Could you check a few things on this model? Use its own coordinates, in mm. Face numbers are marked on the shaded views. A direction names the side the tool comes from. Give positions to 0.01 mm unless a question says otherwise; leave off trailing zeros. Write each loop counter-clockwise with the first axis right and the second up, starting at its lowest first coordinate (ties: lowest second). Pieces come first, ordered by that corner, then holes. Notation, with made-up numbers: M 75.5,88.5 L 134.5,88.5 A29 cw 134.5,115.5 Z; hole C 9.25,66 d3. An arc over 180 degrees is marked long. One line per item, written item: value.
```python
from build123d import *

# Parameters (mm, degrees)
SKETCH1_R           = 1.27
BOSS_EXTRUDE1_DEPTH = 5.08
SKETCH2_R           = 1.5875
BOSS_EXTRUDE2_DEPTH = 12.7


with BuildPart() as part:
    # Sketch1 → Boss-Extrude1 (new body)
    with BuildSketch(Plane(origin=(0, 0, 0), x_dir=(1, 0, 0), z_dir=(0, 1, 0))):
        with BuildLine():
            Line((-10.810601837, 6.664899694), (-3.175, 19.05))
            Line((-3.175, 19.05), (3.175, 19.05))
            Line((3.175, 19.05), (10.810601837, 6.664899694))
            ThreePointArc((10.810601837, 6.664899694), (0, -12.7), (-10.810601837, 6.664899694))
        make_face()
        with Locations(Location((0, 7.62, 0), (0, 0, 270))):
            Circle(SKETCH1_R, mode=Mode.SUBTRACT)
        with Locations(Location((7.62, 0, 0), (0, 0, 270))):
            Circle(SKETCH1_R, mode=Mode.SUBTRACT)
        with Locations(Location((0, -7.62, 0), (0, 0, 270))):
            Circle(SKETCH1_R, mode=Mode.SUBTRACT)
        with Locations(Location((-7.62, 0, 0), (0, 0, 270))):
            Circle(SKETCH1_R, mode=Mode.SUBTRACT)
    extrude(amount=BOSS_EXTRUDE1_DEPTH)

    # Sketch2 → Boss-Extrude2 (add)
    with BuildSketch(Plane(origin=(0, 0, -19.05), x_dir=(-1, 0, 0), z_dir=(0, 0, -1))):
        with Locations((0, 2.54)):
            Circle(SKETCH2_R)
    extrude(amount=BOSS_EXTRUDE2_DEPTH)


solid = part.part
```
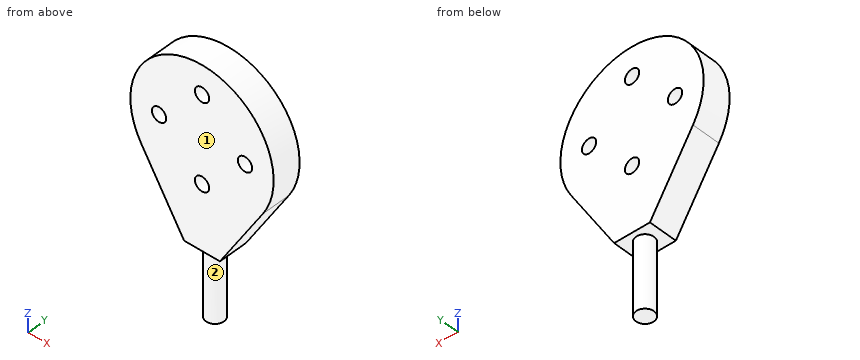
1) If we section it at D-D, the plane x = 7.62: Write out the boundary of the cut face in (y, z), then the cut area to 3 significant figures.
Outcome:
outline: M 0,-11.84 L 5.08,-11.84 L 5.08,-1.27 L 0,-1.27 Z; M 0,1.27 L 5.08,1.27 L 5.08,10.16 L 0,10.16 Z
area: 98.9 mm^2
2) If we section it at A-A, the plane z = 7.62: Write out the boundary of the cut face in (x, y).
Outcome:
outline: M -10.16,0 L -1.27,0 L -1.27,5.08 L -10.16,5.08 Z; M 1.27,0 L 10.16,0 L 10.16,5.08 L 1.27,5.08 Z
3) If we section it at C-C, the plane y = 2.54: Give the number of separate pieces and of enclosed holes in the cut face, then the cut area to 3 significant figures.
Outcome:
separate pieces: 1
enclosed holes: 4
area: 608 mm^2
4) Please list where these lines run through material, in increasing order: L1, parallel to Z at x = 0.5, y = 2.35; L2, parallel to Z at x = -0.75, y = 2.5; L3, parallel to X at y = 2.15, z = 7.62. Write a range as from..to.
Outcome:
L1: z = -31.75..-8.79, -6.45..6.45, 8.79..12.69
L2: z = -31.75..-8.64, -6.6..6.6, 8.64..12.68
L3: x = -10.16..-1.27, 1.27..10.16
5) I'm going to push a flat-ended pin straight in: pin 1 (2 mm diameter, centred on y = 4, z = -11, fed in from +X). Where does the tip first touch, or does it pass through?
Outcome:
pin 1: stops at x = 8.75
6) On a 3-axis mill with a long thin cutter (end or side, diameter ignored), from which of +Z, -Z, +X, -X, +Y, -Y can I reach the whole of each face in a straight line? I mean the marked faces 1 and 2. Say none if no direction works.
Outcome:
face 1: +Z, -Z, +X, -X, -Y
face 2: -Z
7) If we section it at B-B, the plane x = 0: Write out the boundary of the cut face in (y, z).
Outcome:
outline: M 0,-19.05 L 0.95,-19.05 L 0.95,-31.75 L 4.13,-31.75 L 4.13,-19.05 L 5.08,-19.05 L 5.08,-8.89 L 0,-8.89 Z; M 0,-6.35 L 5.08,-6.35 L 5.08,6.35 L 0,6.35 Z; M 0,8.89 L 5.08,8.89 L 5.08,12.7 L 0,12.7 Z
